```python
from build123d import *

# Parameters (mm, degrees)
BOX005_W                = 2
BOX005_H                = 10
BOX005_DEPTH            = 10
CYLINDER029_R           = 9.299038
CYLINDER029_DEPTH       = 10
CYLINDER030_R           = 11.299038
CYLINDER030_DEPTH       = 5
CYLINDER032_R           = 1.25
CYLINDER032_DEPTH       = 5
CYLINDER032_ROLL_ANGLE  = 90
CYLINDER031_R           = 1.25
CYLINDER031_DEPTH       = 5
CYLINDER031_ROLL_ANGLE  = 90
BOX003_W                = 20
BOX003_H                = 2.4
BOX003_DEPTH            = 5
CYLINDER033_R           = 1.5
CYLINDER033_DEPTH       = 10
CYLINDER033_PITCH_ANGLE = 90
BOX004_W                = 8
BOX004_H                = 8
BOX004_DEPTH            = 5


with BuildPart() as quader004:
    # Box005 → Box005 (new body)
    with BuildSketch(Plane(origin=(-1, -19, -1), x_dir=(1, 0, 0), z_dir=(0, 0, 1))):
        with Locations((1, 5)):
            Rectangle(BOX005_W, BOX005_H)
    extrude(amount=BOX005_DEPTH)


with BuildPart() as zylinder027:
    # Cylinder029 → Cylinder029 (new body)
    with BuildSketch(Plane.XY):
        Circle(CYLINDER029_R)
    extrude(amount=CYLINDER029_DEPTH)


with BuildPart() as cut043:
    # Cylinder030 → Cylinder030 (new body)
    with BuildSketch(Plane.XY):
        Circle(CYLINDER030_R)
    extrude(amount=CYLINDER030_DEPTH)

    # Cut043: cut Zylinder027
    add(zylinder027.part, mode=Mode.SUBTRACT)


with BuildPart() as zylinder030:
    # Cylinder032 → Cylinder032 (new body)
    with BuildSketch(Plane.XY):
        Circle(CYLINDER032_R)
    extrude(amount=CYLINDER032_DEPTH)


with BuildPart() as zylinder030_1:
    # Cylinder032 roll: moved
    add(zylinder030.part.rotate(Axis((0, 0, 0), (1, 0, 0)), CYLINDER032_ROLL_ANGLE))


with BuildPart() as zylinder030_2:
    # Cylinder032 placement: moved
    add(zylinder030_1.part.moved(Location((-5, 14, 2.5))))


with BuildPart() as zylinder029:
    # Cylinder031 → Cylinder031 (new body)
    with BuildSketch(Plane.XY):
        Circle(CYLINDER031_R)
    extrude(amount=CYLINDER031_DEPTH)


with BuildPart() as zylinder029_1:
    # Cylinder031 roll: moved
    add(zylinder029.part.rotate(Axis((0, 0, 0), (1, 0, 0)), CYLINDER031_ROLL_ANGLE))


with BuildPart() as zylinder029_2:
    # Cylinder031 placement: moved
    add(zylinder029_1.part.moved(Location((5, 14, 2.5))))


with BuildPart() as cut045:
    # Box003 → Box003 (new body)
    with BuildSketch(Plane(origin=(-10, 9.299038, 0), x_dir=(1, 0, 0), z_dir=(0, 0, 1))):
        with Locations((10, 1.2)):
            Rectangle(BOX003_W, BOX003_H)
    extrude(amount=BOX003_DEPTH)

    # Cut044: cut Zylinder029
    add(zylinder029_2.part, mode=Mode.SUBTRACT)

    # Cut045: cut Zylinder030
    add(zylinder030_2.part, mode=Mode.SUBTRACT)


with BuildPart() as zylinder031:
    # Cylinder033 → Cylinder033 (new body)
    with BuildSketch(Plane.XY):
        Circle(CYLINDER033_R)
    extrude(amount=CYLINDER033_DEPTH)


with BuildPart() as zylinder031_1:
    # Cylinder033 pitch: moved
    add(zylinder031.part.rotate(Axis((0, 0, 0), (0, 1, 0)), CYLINDER033_PITCH_ANGLE))


with BuildPart() as zylinder031_2:
    # Cylinder033 placement: moved
    add(zylinder031_1.part.moved(Location((-5, -14, 2.5))))


with BuildPart() as obj1:
    # Box004 → Box004 (new body)
    with BuildSketch(Plane(origin=(-4, -17.299038, 0), x_dir=(1, 0, 0), z_dir=(0, 0, 1))):
        with Locations((4, 4)):
            Rectangle(BOX004_W, BOX004_H)
    extrude(amount=BOX004_DEPTH)

    # Cut046: cut Zylinder031
    add(zylinder031_2.part, mode=Mode.SUBTRACT)

    # Fusion003: union Cut043, Cut045
    add(cut043.part)
    add(cut045.part)

    # Cut047: cut Quader004
    add(quader004.part, mode=Mode.SUBTRACT)


solid = obj1.part
```
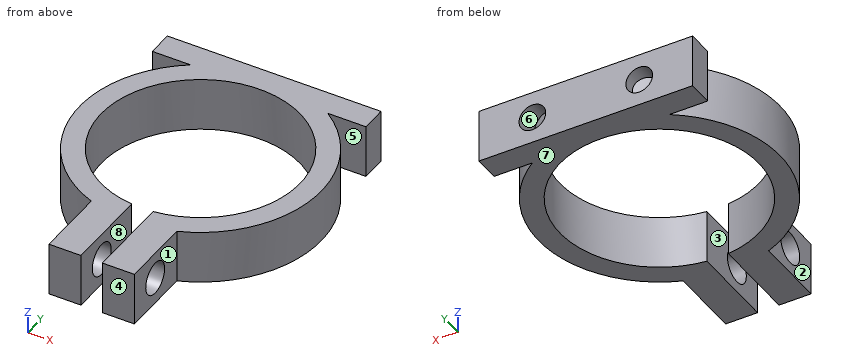
Work out the finished part from the listing and answer in its coordinate system (mm). Face numbers are marked on the shaded views. A direction names the side the tool comes from. Coordinates: 2 decimals unless noted, no trailing zeros. Loops run counter-clockwise (first coordinate to the right, second up) from the corner with the lowest first, then second, coordinate; pieces in that order, holes last. Notation, with made-up numbers: (35.25, -31.5) -> (67.25, -31.5) arc R9 ccw to (67.25, -19.5) -> close; hole circle Ø1 at (-27, 39). An arc over 180 degrees is marked (long way). Answer as CSV lines item,"result".
Q1. For a pull along Z with two mould halves and no side action, classify the marked faces 6, 7 and 8 as +Z half, -Z half, draft (parallel to the pull), parting line (faces both ways), or undercut.
Findings:
face 6,"undercut"
face 7,"-Z half"
face 8,"draft"
Q2. Find the intervals of material crossed by probe 1 along X at (y, z) = (-16, 4.15); probe 2 along Z at (x, y) = (-5, 10.35); probe 3 along Y at (x, z) = (-2.95, 2.5), in increasing order.
Findings:
probe 1,"x = -4 to -1, 1 to 4"
probe 2,"z = 0 to 1.25, 3.75 to 5"
probe 3,"y = -17.3 to -15.5, -12.5 to -8.82, 8.82 to 11.7"
Q3. The part is cut by section C-C on y = -14. Write down the section's boundary in (x, z), and give its area (3 significant figures).
Findings:
outline,"(-4, 0) -> (-1, 0) -> (-1, 1) -> (-4, 1) -> close; (-4, 4) -> (-1, 4) -> (-1, 5) -> (-4, 5) -> close; (1, 0) -> (4, 0) -> (4, 1) -> (1, 1) -> close; (1, 4) -> (4, 4) -> (4, 5) -> (1, 5) -> close"
area,"12.0 mm²"
Q4. Each of these flat-tipped pins is pushed along its axis until it touches: pin 1 (2.5 mm diameter, centred on y = -11.5, z = 3.5, fed in from -X); pin 2 (3 mm diameter, centred on y = 5, z = 4.5, fed in from +X); pin 3 (2.5 mm diameter, centred on y = 10, z = 3, fed in from +X). Where does it stop, or does it pass through?
Findings:
pin 1,"stops at x = -4.75"
pin 2,"stops at x = 10.74"
pin 3,"stops at x = 10"
Q5. The part is cut by section A-A on y = 0. Write down the section's boundary in (x, z), and give its area (3 significant figures).
Findings:
outline,"(-11.3, 0) -> (-9.3, 0) -> (-9.3, 5) -> (-11.3, 5) -> close; (9.3, 0) -> (11.3, 0) -> (11.3, 5) -> (9.3, 5) -> close"
area,"20.0 mm²"
Q6. The part is cut by section B-B on x = 1.75. Write down the section's boundary in (y, z), and give its area (3 significant figures).
Findings:
outline,"(-17.3, 0) -> (-9.13, 0) -> (-9.13, 5) -> (-17.3, 5) -> close; (9.13, 0) -> (11.7, 0) -> (11.7, 5) -> (9.13, 5) -> close; hole circle Ø3 at (-14, 2.5)"
area,"46.6 mm²"
Q7. A tool of negligible diameter and unlimited length cuts with its end or side. For the marked faces 1, 2, 3, 4 and 5, from which of +Z, -Z, +X, -X, +Y, -Y can it reach the whole face along a straight path? Write none if from no direction.
Findings:
face 1,"+Z, -Z, +X, -Y"
face 2,"+Z, -Z, -X, -Y"
face 3,"+Z, -Z, -Y"
face 4,"+Z, -Z, +X, -X, -Y"
face 5,"+Z, -Z, +X"
Q8. The part is cut by section D-D on z = 4.3. Write down the section's boundary in (x, y), and give its area (3 significant figures).
Findings:
outline,"(-10, 9.3) -> (-6.42, 9.3) arc R11.3 ccw to (-4, -10.57) -> (-4, -17.3) -> (-1, -17.3) -> (-1, -9.25) arc R9.3 cw (long way) to (1, -9.25) -> (1, -17.3) -> (4, -17.3) -> (4, -10.57) arc R11.3 ccw to (6.42, 9.3) -> (10, 9.3) -> (10, 11.7) -> (-10, 11.7) -> close"
area,"194 mm²"
